from build123d import *

# Parameters (mm, degrees)
SKETCH_1_R                 = 35
SKETCH_1_R_2               = 2.5
EXTRUDE_1_DEPTH            = 5
EXTRUDE_2_DEPTH            = 30
EXTRUDE_3_DEPTH            = 2.5
PATTERN_LINEAR_1_COUNT     = 2
PATTERN_LINEAR_1_PITCH     = 25
PATTERN_LINEAR_1_COL_COUNT = 2
PATTERN_LINEAR_1_COL_PITCH = 25
MIRROR_1_COPY_1_DEPTH      = 2.5
MIRROR_1_COPY_2_DEPTH      = 2.5
CUT_EXTRUDE_1_REACH        = 56.166
SKETCH_5_R                 = 5.5
SKETCH_6_R                 = 1.5
CUT_EXTRUDE_2_DEPTH        = 71.151518001


with BuildPart() as part:
    # 草圖1 → 填料-伸長1 (new body)
    with BuildSketch(Plane(origin=(0, 0, 0), x_dir=(1, 0, 0), z_dir=(0, 1, 0))):
        with Locations(Location((0, 0, 0), (0, 0, 270))):
            Circle(SKETCH_1_R)
        with Locations(Location((0, 25, 0), (0, 0, 270))):
            Circle(SKETCH_1_R_2, mode=Mode.SUBTRACT)
        with Locations(Location((25, 0, 0), (0, 0, 270))):
            Circle(SKETCH_1_R_2, mode=Mode.SUBTRACT)
        with Locations(Location((0, -25, 0), (0, 0, 270))):
            Circle(SKETCH_1_R_2, mode=Mode.SUBTRACT)
        with Locations(Location((-25, 0, 0), (0, 0, 270))):
            Circle(SKETCH_1_R_2, mode=Mode.SUBTRACT)
    extrude(amount=EXTRUDE_1_DEPTH)

    # 草圖3 → 填料-伸長2 (add, symmetric)
    with BuildSketch(Plane(origin=(0, 0, 0), x_dir=(-0.7071067811865477, 0, -0.7071067811865474), z_dir=(0.7071067811865474, 0, -0.7071067811865477))):
        Polygon((15.25, 5), (-15.25, 5), (-15.25, 27), (-10.25, 27), (-10.25, 7), (10.25, 7), (10.25, 27), (15.25, 27), align=None)
    extrude(amount=EXTRUDE_2_DEPTH, both=True)

    # 草圖4 → 填料-伸長3 (add, symmetric)
    with BuildSketch(Plane(origin=(0, 0, 0), x_dir=(-0.7071067811865477, 0, -0.7071067811865474), z_dir=(0.7071067811865474, 0, -0.7071067811865477))):
        Polygon((-15.25, 12), (-15.25, 5), (-20.25, 5), align=None)
    extrude_3 = extrude(amount=EXTRUDE_3_DEPTH, both=True)

    # 直線複製排列1: 填料-伸長3 ×2
    with Locations(*[Vector(-0.7071067811865474, 0, 0.7071067811865478) * (i * PATTERN_LINEAR_1_PITCH) for i in range(1, PATTERN_LINEAR_1_COUNT)]):
        add(extrude_3)

    # 直線複製排列1 col: 填料-伸長3 ×2
    with Locations(*[Vector(0.7071067811865474, 0, -0.7071067811865478) * (i * PATTERN_LINEAR_1_COL_PITCH) for i in range(1, PATTERN_LINEAR_1_COL_COUNT)]):
        add(extrude_3)

    # 鏡射1: 填料-伸長3 across plane
    add(extrude_3.mirror(Plane(origin=(0, 0, 0), x_dir=(-0.7071067811865474, 0, 0.7071067811865477), z_dir=(0.7071067811865477, 0, 0.7071067811865474))))

    # 鏡射1 copy 1 sketch → 鏡射1 copy 1 (add, symmetric)
    with BuildSketch(Plane(origin=(-17.67766953, 0, 17.67766953), x_dir=(0.7071067811865477, 0, 0.7071067811865474), z_dir=(0.7071067811865474, 0, -0.7071067811865477))):
        Polygon((-15.25, -12), (-15.25, -5), (-20.25, -5), align=None)
    extrude(amount=MIRROR_1_COPY_1_DEPTH, both=True)

    # 鏡射1 copy 2 sketch → 鏡射1 copy 2 (add, symmetric)
    with BuildSketch(Plane(origin=(17.67766953, 0, -17.67766953), x_dir=(0.7071067811865477, 0, 0.7071067811865474), z_dir=(0.7071067811865474, 0, -0.7071067811865477))):
        Polygon((-15.25, -12), (-15.25, -5), (-20.25, -5), align=None)
    extrude(amount=MIRROR_1_COPY_2_DEPTH, both=True)

    # 除料-伸長1: up to this face of the body (flat: up to its plane)
    cut_extrude_1_end = Plane(part.part.faces().sort_by_distance((-9.01561146, 27, -9.01561146))[0])
    # 草圖5 → 除料-伸長1 (cut, up to the picked face)
    with BuildSketch(Plane(origin=(0, 5, 0), x_dir=(1, 0, 0), z_dir=(0, 1, 0)), mode=Mode.PRIVATE) as cut_extrude_1_sk1:
        with Locations((0, 25)):
            Circle(SKETCH_5_R)
    cut_extrude_1_tool1 = split(extrude(cut_extrude_1_sk1.sketch, amount=CUT_EXTRUDE_1_REACH, mode=Mode.PRIVATE), bisect_by=cut_extrude_1_end, keep=Keep.BOTH, mode=Mode.PRIVATE)
    # 草圖5 → 除料-伸長1 (cut, up to the picked face)
    with BuildSketch(Plane(origin=(0, 5, 0), x_dir=(1, 0, 0), z_dir=(0, 1, 0)), mode=Mode.PRIVATE) as cut_extrude_1_sk2:
        with Locations((-25, 0)):
            Circle(SKETCH_5_R)
    cut_extrude_1_tool2 = split(extrude(cut_extrude_1_sk2.sketch, amount=CUT_EXTRUDE_1_REACH, mode=Mode.PRIVATE), bisect_by=cut_extrude_1_end, keep=Keep.BOTH, mode=Mode.PRIVATE)
    # 草圖5 → 除料-伸長1 (cut, up to the picked face)
    with BuildSketch(Plane(origin=(0, 5, 0), x_dir=(1, 0, 0), z_dir=(0, 1, 0)), mode=Mode.PRIVATE) as cut_extrude_1_sk3:
        with Locations((0, -25)):
            Circle(SKETCH_5_R)
    cut_extrude_1_tool3 = split(extrude(cut_extrude_1_sk3.sketch, amount=CUT_EXTRUDE_1_REACH, mode=Mode.PRIVATE), bisect_by=cut_extrude_1_end, keep=Keep.BOTH, mode=Mode.PRIVATE)
    # 草圖5 → 除料-伸長1 (cut, up to the picked face)
    with BuildSketch(Plane(origin=(0, 5, 0), x_dir=(1, 0, 0), z_dir=(0, 1, 0)), mode=Mode.PRIVATE) as cut_extrude_1_sk4:
        with Locations((25, 0)):
            Circle(SKETCH_5_R)
    cut_extrude_1_tool4 = split(extrude(cut_extrude_1_sk4.sketch, amount=CUT_EXTRUDE_1_REACH, mode=Mode.PRIVATE), bisect_by=cut_extrude_1_end, keep=Keep.BOTH, mode=Mode.PRIVATE)
    add(cut_extrude_1_tool1.solids().sort_by(Axis((0, 5, -25), (0, 1, 0)))[0], mode=Mode.SUBTRACT)
    add(cut_extrude_1_tool2.solids().sort_by(Axis((-25, 5, 0), (0, 1, 0)))[0], mode=Mode.SUBTRACT)
    add(cut_extrude_1_tool3.solids().sort_by(Axis((0, 5, 25), (0, 1, 0)))[0], mode=Mode.SUBTRACT)
    add(cut_extrude_1_tool4.solids().sort_by(Axis((25, 5, 0), (0, 1, 0)))[0], mode=Mode.SUBTRACT)

    # 草圖6 → 除料-伸長2 (cut, through all)
    with BuildSketch(Plane(origin=(-10.783378413, 0, -10.783378413), x_dir=(-0.7071067811865474, 0, 0.7071067811865477), z_dir=(-0.7071067811865477, 0, -0.7071067811865474))):
        with Locations((0, 17)):
            Circle(SKETCH_6_R)
        with Locations((-26.5, 17)):
            Circle(SKETCH_6_R)
        with Locations((26.5, 17)):
            Circle(SKETCH_6_R)
    extrude(amount=-CUT_EXTRUDE_2_DEPTH, mode=Mode.SUBTRACT)


solid = part.part
Input: part model. Units: mm. Frame: model coordinates. A direction names the side the tool comes from. Coordinates: 2 decimals unless noted, no trailing zeros. Order: outer loops, then holes, each group sorted by start corner. A loop starts at its lowest first (then second) coordinate and runs counter-clockwise, first axis right, second up. Notation, with made-up numbers: M 58,66.25 L 117,66.25 A25 cw 117,97.25 Z; hole C 60,59 d2. An arc over 180 degrees is marked long. Write item = value, one per line. Start each with the question number.
(1) Line query: line 1 along Z through (x, y) = (13, 10); line 2 along Y through (x, z) = (-10, 27.5); line 3 along Y through (x, z) = (12.5, -3). Output: solid intervals per line, ascending. Write a range as [from, to].
(2) Pull-direction query (Z, two-part tool) for faces 5 (the flat face through (-23.76, 6.376, 18.666)), 6 (the flat face through (18.666, 6.376, -23.76)), 7 (the cylindrical face through (-4.25, 15.85, 21.51)); classes: released by +Z, released by -Z, zero draft, split by the parting line, or undercut.
(3) Section B-B on z = 0. Output: boundary loops of the cut face in (x, y), and give its area (3 significant figures).
(4) Reachability of faces 1 (the flat face through (31.19, 6.99, -7.7)), 2 (the flat face through (-9.973, 6.993, -13.508)), 3 (the flat face through (7.545, 19.362, 6.951)), 4 (the flat face through (-7.7, 6.99, 31.19)) from +Z, -Z, +X, -X, +Y, -Y: full face, straight path, thin tool, end or side. Return the list, or none.
(5) Section A-A on y = 13.25. Output: boundary loops of the cut face in (x, z), and give its area (3 significant figures).
(6) First-contact query: P1, Ø8, axis at x = 0, z = 25, coming from the +Y side; P2, Ø1, axis at y = 9, z = -8, coming from the -X side; P3, Ø5, axis at x = 9.5, z = 25.5, coming from the -Y side; P4, Ø6, axis at y = 23, z = -27, coming from the -X side. Flat tips, straight axial feed; report the tip coordinate or a pass-through.
(7) Section C-C on x = 0. Output: boundary loops of the cut face in (y, z).
(8) Section D-D on x = 21. Output: boundary loops of the cut face in (y, z), and give its area (3 significant figures).
Result set:
q1.line_1 = [-29.43, -27.5], [1.5, 8.57], [9.46, 10.59]
q1.line_2 = [0, 15.5], [18.5, 27]
q1.line_3 = [0, 7]
q2.face_5 = released by +Z
q2.face_6 = released by -Z
q2.face_7 = undercut
q3.outline = M -35,0 L -27.5,0 L -27.5,5 L -35,5 Z; M -22.5,0 L 22.5,0 L 22.5,5 L 19.5,5 L 19.5,27 L 14.5,27 L 14.5,7 L -14.5,7 L -14.5,27 L -19.5,27 L -19.5,5 L -22.5,5 Z; M 27.5,0 L 35,0 L 35,5 L 27.5,5 Z
q3.area = 578 mm²
q4.face_1 = +X, +Y
q4.face_2 = -Z, +Y
q4.face_3 = +Y
q4.face_4 = +Z, +Y
q5.outline = M -32,10.43 L -26.77,5.21 A5.5 cw -19.79,-1.77 L -1.77,-19.79 A5.5 cw 5.21,-26.77 L 10.43,-32 L 13.97,-28.46 L -28.46,13.97 Z; M -13.97,28.46 L 28.46,-13.97 L 32,-10.43 L 26.77,-5.21 A5.5 cw 19.79,1.77 L 1.77,19.79 A5.5 cw -5.21,26.77 L -10.43,32 Z
q5.area = 513 mm²
q6.P1 = 5
q6.P2 = -14.07
q6.P3 = 0
q6.P4 = 5.21
q7.outline = M 0,-35 L 5,-35 L 5,-27.5 L 0,-27.5 Z; M 0,-22.5 L 5,-22.5 L 5,-19.5 L 27,-19.5 L 27,-14.5 L 7,-14.5 L 7,14.5 L 27,14.5 L 27,19.5 L 5,19.5 L 5,22.5 L 0,22.5 Z; M 0,27.5 L 5,27.5 L 5,35 L 0,35 Z
q8.outline = M 0,-28 L 5,-28 L 5,-21.43 L 7,-21.43 L 7,-6.5 L 27,-6.5 L 27,-3.77 L 5,-3.77 L 5,28 L 0,28 Z
q8.area = 370 mm²
